Autodesk Inventor part; units mm, degrees
ref_plane "Work Plane1" through (0, 0, 0) normal (0, -0.866, 0.5) x (1, 0, 0)
ref_plane "YZ Plane" through (0, 0, 0) normal (1, 0, 0) x (0, 1, 0)
ref_plane "XZ Plane" through (0, 0, 0) normal (0, 1, 0) x (-1, 0, 0)
ref_plane "Work Plane1" through (0, 0, 0) normal (0, -0.866, 0.5) x (1, 0, 0)
sketch "Sketch1" plane through (0, 0, 0) normal (0, -0.866, 0.5) x (1, 0, 0)
  circle A0 centre (0, 0) radius 97 construction
  dimension "d1" = 194
sketch "Sketch2" plane through (0, 0, 0) normal (0, 1, 0) x (-1, 0, 0)
  point P0 (0, 0)
sketch "Sketch3" plane through (0, 0, 0) normal (0, 0, 1) x (1, 0, 0)
  ellipse E0 centre (0, 0) end of major axis (97, 0) minor radius 48.5 construction
  circle A0 centre (0, -31.5) radius 17
  line L0 (0, -31.5) -> (44.8665, -31.5)
  line L1 (0, -43) -> (44.8665, -43) construction
  line L2 (0, -31.5) -> (-44.8665, -31.5)
  line L3 (0, -43) -> (-44.8665, -43) construction
  line L4 (44.8665, -43) -> (44.8665, -31.5)
  line L5 (-44.8665, -43) -> (-44.8665, -31.5)
  arc A1 (-44.8665, -43) -> (44.8665, -43) centre (0, 137.25) ccw
  dimension "d3" = 11.5
revolve "Revolution1" add sketch "Sketch3" angle 360 about axis through (0, -31.5, 0) along (1, 0, 0) picked at (1.261, -42.6913) contours L0 L4 A1 A0 | A0 L2 L0 | A0 A1 L5 L2
sketch "Sketch4" plane through (-44.8665, -31.5, 0) normal (-1, 0, 0) x (0, 0, 1)
  circle A0 centre (0, 0) radius 9.5
  point P0 (0, 31.5)
  dimension "d5" = 19
extrude "Extrusion1" cut sketch "Sketch4" against normal blind 6
sketch "Sketch5" plane through (-38.8665, -31.5, 0) normal (-1, 0, 0) x (0, 0, 1)
  circle A0 centre (0, 0) radius 4
  point P0 (0, 31.5)
  dimension "d8" = 8
extrude "Extrusion2" cut sketch "Sketch5" against normal blind 100
sketch "Sketch6" plane through (44.8665, -31.5, 0) normal (1, 0, 0) x (0, 0, -1)
  circle A0 centre (0, 0) radius 4
  circle A1 centre (0, 0) radius 9.5
  point P0 (0, 31.5)
extrude "Extrusion3" cut sketch "Sketch6" against normal blind 6
properties part number "roller test"
Design review of the part built by this model. Coordinates are the model's own, in mm. A direction names the side the tool comes from. Round coordinates to 2 decimals unless told otherwise and drop trailing zeros. One line per question, with ' | ' between items.
Item 1: Wall thickness on line 1 (X direction, y = -39, z = -5.5); line 2 (Z direction, x = 9, y = -31); line 3 (Z direction, x = 4, y = -29.5): over which ranges is each line inside the solid? List them lowest first. Write a range as [from, to].
Checks:
line 1: [-38.87, 38.87] | line 2: [-16.77, -3.97], [3.97, 16.77] | line 3: [-16.84, -3.46], [3.46, 16.84]
Item 2: Machinability: for faces 1 (the face through (41.908, -28.646, -9.061)), 2 (the face through (-41.908, -28.646, 9.061)), 3 (the face through (-44.866, -27, -9)), which of the approach directions +Z, -Z, +X, -X, +Y, -Y give a long, thin tool a straight path to every point of the face, cutting with its end or side? Answer none if there is none.
Checks:
face 1: +X | face 2: -X | face 3: +Z, -Z, -X, +Y, -Y
Item 3: Draft analysis for pull direction Y (two halves, no side actions). For faces 4 (the face through (44.866, -27, -9)), 5 (the face through (38.866, -36, 0)), state which applies: +Y half, -Y half, draft (parallel to the pull), parting line (faces both ways), or undercut.
Checks:
face 4: draft | face 5: undercut
Item 4: For P1, Ø15, axis at y = -33, z = 0.5, coming from the +X side; P2, Ø2, axis at x = 11.5, z = -8, coming from the -Y side (3 decimals); P3, Ø4, axis at x = 27, z = 7.5, coming from the -Y side; P4, Ø5, axis at y = -31.5, z = 0, coming from the -X side, all flat-tipped, find the tip position at first contact; note any pin that passes through.
Checks:
P1: x = 38.87 | P2: y = -46.605 | P3: y = -45.54 | P4: through
